Geometry check sheet. Reference: the model listing, model coordinates, mm. Face numbers are marked on the shaded views. Round coordinates to 2 decimals unless told otherwise and drop trailing zeros. Order: outer loops, then holes, each group sorted by start corner. A loop starts at its lowest first (then second) coordinate and runs counter-clockwise, first axis right, second up. Notation, with made-up numbers: (-4.5, -8.5) - (24.5, -8.5) arc R18 ccw to (24.5, 2.5) - close; hole circle Ø8 at (7.5, 54.5). An arc over 180 degrees is marked (long way). Return JSON: item names as keys, results as strings. Group by question number.
Q1. Draft check along X on the marked faces 1, 2 and 3. Enter one of: pulls with the +X half, pulls with the -X half, needs draft (parallel to the pull), parting line crosses it, or undercut.
Q2. Gauge pin test, flat ends, axial feed: pin 1 Ø1.5 at (x, y) = (9, 8) entering from -Z; pin 2 Ø6 at (x, z) = (-8, -2) entering from -Y; pin 3 Ø4 at (x, y) = (9, 4) entering from +Z (3 decimals); pin 4 Ø2 at (y, z) = (4, 4) entering from -X. Record the tip position at first contact, or that the pin passes through.
Q3. Sectioned sample at D-D, the plane z = 15.5. Record the cut outline in (x, y), then the cut area to 3 significant figures.
Q4. Sectioned sample at B-B, the plane z = 0. Record the cut outline in (x, y).
Q5. Sectioned sample at C-C, the plane y = 11. Record the cut outline in (x, z).
Q6. Sectioned sample at A-A, the plane x = 3.5. Record the cut outline in (y, z), then the cut area to 3 significant figures.
Q7. Material ranges on line 1 along X through (y, z) = (5.25, -6); line 2 along X through (y, z) = (9.5, -4); line 3 along Z through (x, y) = (15, 2.5), recorded low to high.
```python
from build123d import *

# Parameters (mm, degrees)
SKETCH1_R           = 20
SKETCH1_R_2         = 12.5
BOSS_EXTRUDE1_DEPTH = 12
CUT_EXTRUDE1_DEPTH  = 62


with BuildPart() as part:
    # Sketch1 → Boss-Extrude1 (new body)
    with BuildSketch(Plane(origin=(0, 0, 0), x_dir=(1, 0, 0), z_dir=(0, 1, 0))):
        with Locations(Location((0, 0, 0), (0, 0, 270))):
            Circle(SKETCH1_R)
        with Locations(Location((0, 0, 0), (0, 0, 270))):
            Circle(SKETCH1_R_2, mode=Mode.SUBTRACT)
    extrude(amount=BOSS_EXTRUDE1_DEPTH)

    # Sketch3 → Cut-Extrude1 (cut)
    with BuildSketch(Plane.XY.offset(20)):
        with BuildLine():
            ThreePointArc((0, 9), (-3, 6), (0, 3))
            Line((0, 3), (0, 9))
        make_face()
        with BuildLine():
            Line((0, 9), (0, 3))
            ThreePointArc((0, 3), (2.121320344, 3.878679656), (3, 6))
            ThreePointArc((3, 6), (2.121320344, 8.121320344), (0, 9))
        make_face()
    extrude(amount=-CUT_EXTRUDE1_DEPTH, mode=Mode.SUBTRACT)


solid = part.part
```
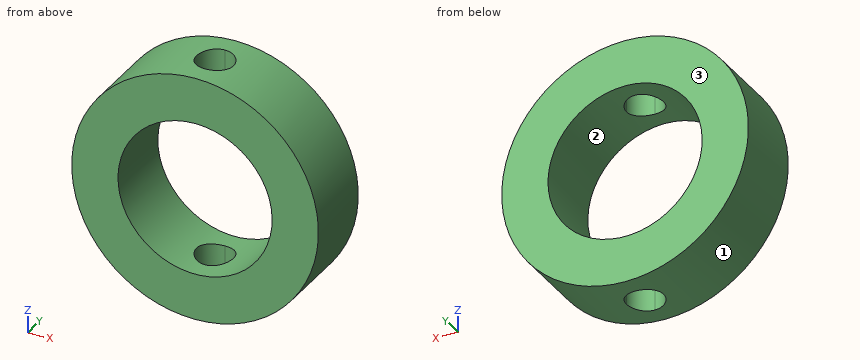
Reply:
{
 "1": {"face 1": "parting line crosses it", "face 2": "undercut", "face 3": "needs draft"},
 "2": {"pin 1": "z = -18.22", "pin 2": "through", "pin 3": "z = 18.735", "pin 4": "x = -19.77"},
 "3": {"outline": "(-12.64, 0) - (12.64, 0) - (12.64, 12) - (-12.64, 12) - close; hole circle Ø6 at (0, 6)", "area": "275 mm^2"},
 "4": {"outline": "(-20, 0) - (-12.5, 0) - (-12.5, 12) - (-20, 12) - close; (12.5, 0) - (20, 0) - (20, 12) - (12.5, 12) - close"},
 "5": {"outline": "circle Ø40 at (0, 0); hole circle Ø25 at (0, 0)"},
 "6": {"outline": "(0, -19.69) - (12, -19.69) - (12, -12) - (0, -12) - close; (0, 12) - (12, 12) - (12, 19.69) - (0, 19.69) - close", "area": "185 mm^2"},
 "7": {"line 1": "-19.08 to -10.97, 10.97 to 19.08", "line 2": "-19.6 to -11.84, 11.84 to 19.6", "line 3": "-13.23 to 13.23"}
}
